Verification items for the finished model (mm, model axes). Coordinates: 2 decimals unless noted, no trailing zeros. Write each loop counter-clockwise with the first axis right and the second up, starting at its lowest first coordinate (ties: lowest second). Pieces come first, ordered by that corner, then holes. Notation, with made-up numbers: (33, 41) -> (66, 41) arc R9 ccw to (66, 52) -> close; hole circle Ø4 at (49.25, 61). An arc over 180 degrees is marked (long way). Answer in a Markdown table with one row per item.
```python
from build123d import *

# Parameters (mm, degrees)
F0_R     = 1.25
F1_DEPTH = 1
F2_W     = 8
F2_H     = 12
F2_W_2   = 3
F2_H_2   = 4
F3_DEPTH = 1


with BuildPart() as f1:
    # F0 (on Top) → F1 (new body)
    with BuildSketch(Plane.XY):
        with BuildLine():
            Line((1.405504, 3.364061), (-59.594496, 3.364061))
            Line((-59.594496, 3.364061), (-60.094496, 1.364061))
            Line((-60.094496, 1.364061), (-60.094496, -4.635939))
            ThreePointArc((-60.094496, -4.635939), (-58.094496, -6.635939), (-60.094496, -8.635939))
            Line((-60.094496, -8.635939), (-60.094496, -12.811412))
            ThreePointArc((-60.094496, -12.811412), (-58.094496, -14.811412), (-60.094496, -16.811412))
            Line((-60.094496, -16.811412), (-60.094496, -25.811412))
            Line((-60.094496, -25.811412), (-59.094496, -26.811412))
            Line((-59.094496, -26.811412), (71.905504, -26.811412))
            Line((71.905504, -26.811412), (72.905504, -25.811412))
            Line((72.905504, -25.811412), (72.905504, -16.811412))
            ThreePointArc((72.905504, -16.811412), (70.905504, -14.811412), (72.905504, -12.811412))
            Line((72.905504, -12.811412), (72.905504, -8.635939))
            ThreePointArc((72.905504, -8.635939), (70.905504, -6.635939), (72.905504, -4.635939))
            Line((72.905504, -4.635939), (72.905504, 1.133777))
            Line((72.905504, 1.133777), (72.405504, 3.364061))
            Line((72.405504, 3.364061), (2.905504, 3.364061))
            Line((2.905504, 3.364061), (2.905504, 0))
            ThreePointArc((2.905504, 0), (2.155504, -0.547161), (1.405504, 0))
            Line((1.405504, 0), (1.405504, 3.364061))
        make_face()
        with Locations((-57.844496, 1.114061)):
            Circle(F0_R, mode=Mode.SUBTRACT)
        with Locations((70.655504, 1.114061)):
            Circle(F0_R, mode=Mode.SUBTRACT)
    extrude(amount=F1_DEPTH)

    # F2 (on face) → F3 (join)
    with BuildSketch(Plane.XY.offset(1)):
        with Locations((-50.094496, -13.811412)):
            Rectangle(F2_W, F2_H)
        with Locations((-36.094496, -13.811412)):
            Rectangle(F2_W, F2_H)
        with Locations((-22.094496, -13.811412)):
            Rectangle(F2_W, F2_H)
        with Locations((-8.094496, -13.811412)):
            Rectangle(F2_W, F2_H)
        with Locations((62.905504, -13.811412)):
            Rectangle(F2_W, F2_H)
        with Locations((48.905504, -13.811412)):
            Rectangle(F2_W, F2_H)
        with Locations((34.905504, -13.811412)):
            Rectangle(F2_W, F2_H)
        with Locations((20.905504, -13.811412)):
            Rectangle(F2_W, F2_H)
        with Locations((0.405504, -4.311412)):
            Rectangle(F2_W_2, F2_H_2)
    extrude(amount=F3_DEPTH)


solid = f1.part
```
1. Section check B-B, the plane z = 1.45. State how many separate pieces and enclosed holes the cut face has, plus the area to 3 significant figures.
Geometry says:
| item | result |
|---|---|
| separate pieces | 9 |
| enclosed holes | 0 |
| area | 780 mm^2 |
2. Section check A-A, the plane x = 37. Record the boundary of the cut face in (y, z).
Geometry says:
| item | result |
|---|---|
| outline | (-26.81, 0) -> (3.36, 0) -> (3.36, 1) -> (-7.81, 1) -> (-7.81, 2) -> (-19.81, 2) -> (-19.81, 1) -> (-26.81, 1) -> close |
3. Depth check by flat-ended pin: P1, Ø0.5, axis at x = 23, z = 1.5, coming from the +Y side; P2, Ø1, axis at x = -0.5, y = 0, coming from the +Z side; P3, Ø0.8, axis at x = 0.5, z = 1.5, coming from the +Y side. Enter the tip coordinate at first touch or a pass-through.
Geometry says:
| item | result |
|---|---|
| P1 | y = -7.81 |
| P2 | z = 1 |
| P3 | y = -2.31 |
4. Mould release check, pull along X, two halves, no side actions. Record for faces 1 (the cylindrical face through (71.81, 0.64, 0.49)), 2 (the flat face through (-36, -14, 2)), 3 (the cylindrical face through (-59.093, 1.169, 0.493)): released by +X, released by -X, zero draft, split by the parting line, or undercut.
Geometry says:
| item | result |
|---|---|
| face 1 | undercut |
| face 2 | zero draft |
| face 3 | undercut |
5. Section check C-C, the plane x = -3. Record the boundary of the cut face in (y, z).
Geometry says:
| item | result |
|---|---|
| outline | (-26.81, 0) -> (3.36, 0) -> (3.36, 1) -> (-26.81, 1) -> close |
6. Thickness scan on line 1 (Y direction, x = 1, z = 1.2); line 2 (Y direction, x = 36.5, z = 1.05); line 3 (Z direction, x = -31.5, y = -8). Record the ranges inside material, lowest first. Write a range as from..to.
Geometry says:
| item | result |
|---|---|
| line 1 | -6.31..-2.31 |
| line 2 | -19.81..-7.81 |
| line 3 | 0..1 |
